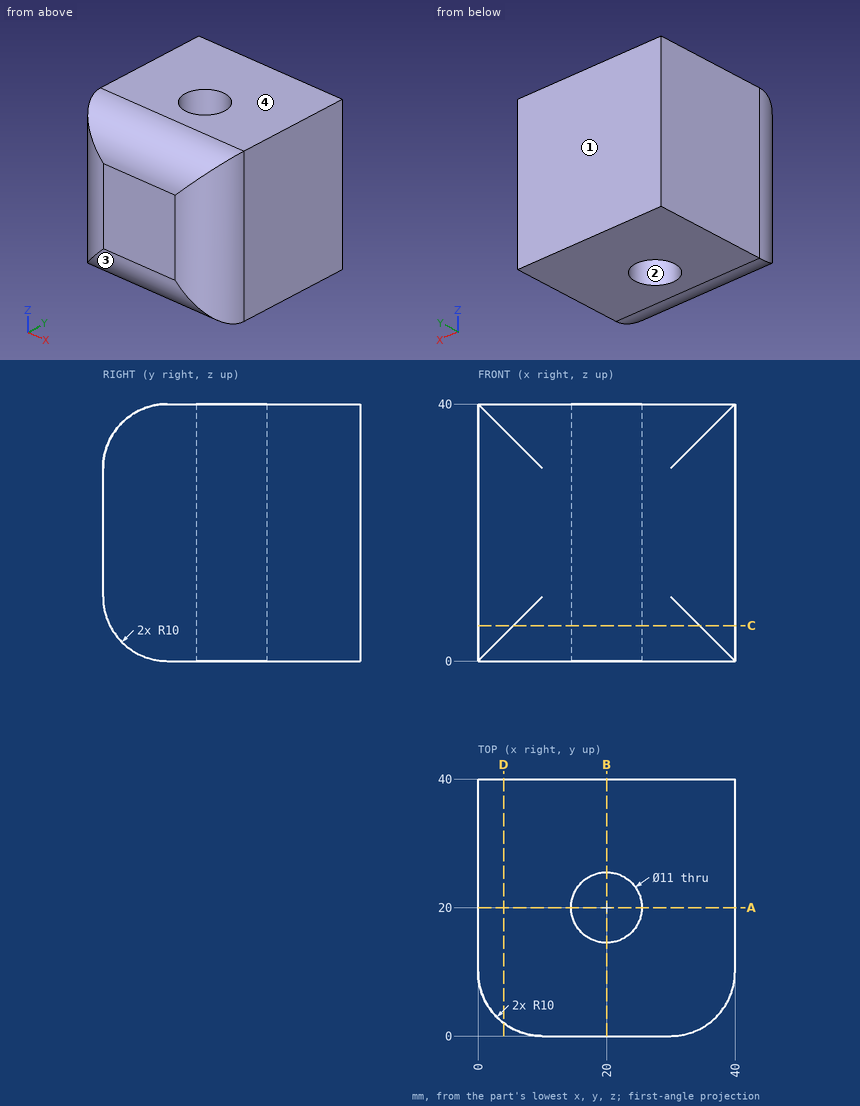
Can you work these out from the drawing? Everything is in mm from the part's minimum corner. Give positions to 0.01 mm unless a question says otherwise; leave off trailing zeros. Loops run counter-clockwise (first coordinate to the right, second up) from the corner with the lowest first, then second, coordinate; pieces in that order, holes last. Notation, with made-up numbers: (45.25, 58.5) -> (94.25, 58.5) arc R27 ccw to (94.25, 76.5) -> close; hole circle Ø5 at (43, 22). An arc over 180 degrees is marked (long way). Return JSON: item names as keys, results as strings.
Q1. I want a section at B-B, the plane x = 20. List the corners of the cut face in (y, z) for me.
Checks:
{"outline": "(0, 10) arc R10 ccw to (10, 0) -> (14.5, 0) -> (14.5, 40) -> (10, 40) arc R10 ccw to (0, 30) -> close; (25.5, 0) -> (40, 0) -> (40, 40) -> (25.5, 40) -> close"}
Q2. I want a section at A-A, the plane y = 20. List the corners of the cut face in (x, z) for me.
Checks:
{"outline": "(0, 0) -> (14.5, 0) -> (14.5, 40) -> (0, 40) -> close; (25.5, 0) -> (40, 0) -> (40, 40) -> (25.5, 40) -> close"}
Q3. We'd pull the mould along Y, two halves only. Please class the marked faces 1, 2, 3 and 4: released by +Y, released by -Y, zero draft, split by the parting line, or undercut.
Checks:
{"face 1": "released by +Y", "face 2": "undercut", "face 3": "released by -Y", "face 4": "zero draft"}
Q4. I want a section at C-C, the plane z = 5.5. List the corners of the cut face in (x, y) for me, then the cut area to 3 significant figures.
Checks:
{"outline": "(0, 10) arc R10 ccw to (5.5, 1.07) -> (34.5, 1.07) arc R10 ccw to (40, 10) -> (40, 40) -> (0, 40) -> close; hole circle Ø11 at (20, 20)", "area": "1,430 mm2"}
Q5. I need wall thicknesses on probe 1 along Y at (x, z) = (20, 12); probe 2 along X at (y, z) = (15.5, 2); probe 3 along X at (y, z) = (23, 31.5). Which ranges of each line are inside material? Lowest first, please.
Checks:
{"probe 1": "y = 0 to 14.5, 25.5 to 40", "probe 2": "x = 0 to 16.84, 23.16 to 40", "probe 3": "x = 0 to 15.39, 24.61 to 40"}
Q6. I want a section at D-D, the plane x = 4. List the corners of the cut face in (y, z) for me, then the cut area to 3 significant figures.
Checks:
{"outline": "(2, 4) arc R10 ccw to (10, 0) -> (40, 0) -> (40, 40) -> (10, 40) arc R10 ccw to (2, 36) -> close", "area": "1,500 mm2"}
Q7. For pin 1 Ø4 at (x, y) = (24.5, 24.5) entering from -Z, with a flat end and sliding along its axis, tell me the tip position at first contact or that it passes through.
Checks:
{"pin 1": "stops at z = 0"}
